Geometry check sheet. Reference: the model listing, model coordinates, mm. Face numbers are marked on the shaded views. A direction names the side the tool comes from. Coordinates: 2 decimals unless noted, no trailing zeros. Order: outer loops, then holes, each group sorted by start corner. A loop starts at its lowest first (then second) coordinate and runs counter-clockwise, first axis right, second up. Notation, with made-up numbers: (53, -7.75) - (109, -7.75) arc R6 ccw to (109, 1.25) - close; hole circle Ø5 at (44, -19.75). An arc over 180 degrees is marked (long way). Put each result on its own line as item: value.
Autodesk Inventor part; units mm, degrees
ref_plane "YZ Plane" through (0, 0, 0) normal (1, 0, 0) x (0, 1, 0)
ref_plane "XZ Plane" through (0, 0, 0) normal (0, 1, 0) x (-1, 0, 0)
ref_plane "XY Plane" through (0, 0, 0) normal (0, 0, 1) x (1, 0, 0)
sketch "Sketch1" plane through (0, 0, 0) normal (0, 0, 1) x (1, 0, 0)
  line L0 (0, 0) -> (1.5, 0)
  line L1 (1.5, 0) -> (1.5, -2.5)
  line L2 (1.5, -2.5) -> (0, -2.5)
  line L3 (0, -2.5) -> (0, 0)
  dimension "d0" = 1.5
  dimension "d1" = 2.5
extrude "Extrusion1" add sketch "Sketch1" along normal blind 10
sketch "Sketch2" plane through (0, 0, 0) normal (0, 1, 0) x (1, 0, 0)
  line L0 (0, -10) -> (1.5, -10)
  line L1 (1.5, 0) -> (1.5, -10)
  line L2 (0, -10) -> (1.5, -10)
  line L3 (1.5, -10) -> (1.5, -8.5)
  line L4 (1.5, -8.5) -> (0, -8.5)
  line L5 (0, -8.5) -> (0, -10)
  point P0 (0, 0)
  dimension "d4" = 1.5
extrude "Extrusion2" add sketch "Sketch2" along normal blind 2
fillet "Fillet1" radius 0.5 1 edges at (1.5, 2, 9.25)
fillet "Fillet2" radius 0.5 1 edges at (0, 2, 9.25)
properties part number "Key"
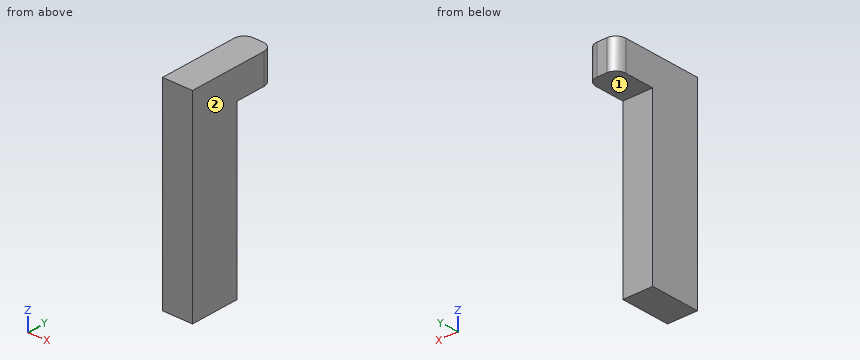
Q1. Access from +Z, -Z, +X, -X, +Y, -Y to the whole of each face (thin tool, end or side, straight path). Record for the marked faces 1 and 2.
Answer block:
face 1: -Z, +X, -X, +Y
face 2: +Z, -Z, +X, +Y, -Y
Q2. Thickness scan on L1, parallel to Y at x = 1.25, z = 6.25; L2, parallel to Z at x = 1.2, y = 1.5; L3, parallel to Y at x = 1.15, z = 9. Record the ranges inside material, lowest first. Write a range as [from, to].
Answer block:
L1: y = [-2.5, 0]
L2: z = [8.5, 10]
L3: y = [-2.5, 1.98]
Q3. Section check D-D on z = 4. Record the boundary of the cut face in (x, y), then the cut area to 3 significant figures.
Answer block:
outline: (0, -2.5) - (1.5, -2.5) - (1.5, 0) - (0, 0) - close
area: 3.75 mm^2
Q4. Depth check by flat-ended pin: pin 1 Ø1 at (y, z) = (-0.5, 6) entering from -X. Enter the tip coordinate at first touch or a pass-through.
Answer block:
pin 1: stops at x = 0
Q5. Section check A-A on z = 9.25. Record the boundary of the cut face in (x, y), then the cut area to 3 significant figures.
Answer block:
outline: (0, -2.5) - (1.5, -2.5) - (1.5, 1.5) arc R0.5 ccw to (1, 2) - (0.5, 2) arc R0.5 ccw to (0, 1.5) - close
area: 6.64 mm^2
Q6. Section check C-C on y = 0.35. Record the boundary of the cut face in (x, z), then the cut area to 3 significant figures.
Answer block:
outline: (0, 8.5) - (1.5, 8.5) - (1.5, 10) - (0, 10) - close
area: 2.25 mm^2
Q7. Section check B-B on x = 1.4. Record the boundary of the cut face in (y, z), then the cut area to 3 significant figures.
Answer block:
outline: (-2.5, 0) - (0, 0) - (0, 8.5) - (1.8, 8.5) - (1.8, 10) - (-2.5, 10) - close
area: 27.7 mm^2
